Source: CAD feature listing. Evaluate the final solid. Frame: model axes, mm. A direction names the side the tool comes from. Coordinates: 2 decimals unless noted, no trailing zeros. Write each loop counter-clockwise with the first axis right and the second up, starting at its lowest first coordinate (ties: lowest second). Pieces come first, ordered by that corner, then holes. Notation, with made-up numbers: (40, 13) -> (57, 13) arc R22 cw to (57, 26) -> close; hole circle Ø10 at (69.5, 45.5). An arc over 180 degrees is marked (long way). Write item = value, one per line.
from build123d import *

# Parameters (mm, degrees)
BOSS_EXTRUDE1_DEPTH = 115.8875
CUT_EXTRUDE1_REACH  = 194.846
SKETCH3_W           = 213.51875
SKETCH3_H           = 129.38125
CUT_EXTRUDE3_DEPTH  = 4.7625
FILLET1_R           = 3.175
CUT_EXTRUDE4_START  = -4.7625
CUT_EXTRUDE4_DEPTH  = 4.7625


with BuildPart() as part:
    # Sketch1 → Boss-Extrude1 (new, symmetric)
    with BuildSketch(Plane.XY):
        Polygon((0, 0), (65.143179844, 139.7), (65.143179844, 124.674619947), (7.006449785, 0), align=None)
    extrude(amount=BOSS_EXTRUDE1_DEPTH, both=True)

    # Sketch2 → Cut-Extrude1 (cut, up to next)
    with BuildSketch(Plane(origin=(0, 0, 0), x_dir=(0, 0, 1), z_dir=(-0.906307787036651, 0.42261826174069705, 0)), mode=Mode.PRIVATE) as cut_extrude1_sk1:
        with BuildLine():
            Line((-98.679, 15.944158686), (-98.679, 128.720158686))
            ThreePointArc((-98.679, 128.720158686), (-98.38142049, 129.438579176), (-97.663, 129.736158686))
            Line((-97.663, 129.736158686), (97.663, 129.736158686))
            ThreePointArc((97.663, 129.736158686), (98.38142049, 129.438579176), (98.679, 128.720158686))
            Line((98.679, 128.720158686), (98.679, 15.944158686))
            ThreePointArc((98.679, 15.944158686), (98.38142049, 15.225738197), (97.663, 14.928158686))
            Line((97.663, 14.928158686), (-97.663, 14.928158686))
            ThreePointArc((-97.663, 14.928158686), (-98.38142049, 15.225738197), (-98.679, 15.944158686))
        make_face()
    cut_extrude1_tool1 = extrude(cut_extrude1_sk1.sketch, amount=-CUT_EXTRUDE1_REACH, mode=Mode.PRIVATE) & part.part
    add(cut_extrude1_tool1.solids().sort_by_distance((30.568891, 65.555199, 0))[0], mode=Mode.SUBTRACT)

    # Sketch3 → Cut-Extrude3 (cut)
    with BuildSketch(Plane(origin=(5.755054448, -2.683625962, 0), x_dir=(0, 0, -1), z_dir=(0.906307787036651, -0.42261826174069717, 0))):
        with Locations((-0.396875, 73.519608686)):
            Rectangle(SKETCH3_W, SKETCH3_H)
    extrude(amount=-CUT_EXTRUDE3_DEPTH, mode=Mode.SUBTRACT)

    # Fillet1
    fillet1_edges = [part.edges().sort_by_distance(p)[0] for p in [
        (7.328198768, 6.32451044, 107.15625),
        (62.007077745, 123.583744812, 107.15625),
        (62.007077745, 123.583744812, -106.3625),
        (7.328198768, 6.32451044, -106.3625),
    ]]
    fillet(fillet1_edges, radius=FILLET1_R)

    # Sketch4 → Cut-Extrude4 (cut)
    with BuildSketch(Plane(origin=(5.755054448, -2.683625962, 0), x_dir=(0, 0, -1), z_dir=(0.906307787036651, -0.42261826174069717, 0)).offset(CUT_EXTRUDE4_START)):
        with BuildLine():
            Line((107.95, 12.003983686), (107.95, 135.035233686))
            ThreePointArc((107.95, 135.035233686), (106.555096045, 138.402829732), (103.1875, 139.797733686))
            Line((103.1875, 139.797733686), (-103.98125, 139.797733686))
            ThreePointArc((-103.98125, 139.797733686), (-107.348846045, 138.402829732), (-108.74375, 135.035233686))
            Line((-108.74375, 135.035233686), (-108.74375, 12.003983686))
            ThreePointArc((-108.74375, 12.003983686), (-107.348846045, 8.636387641), (-103.98125, 7.241483686))
            Line((-103.98125, 7.241483686), (103.1875, 7.241483686))
            ThreePointArc((103.1875, 7.241483686), (106.555096045, 8.636387641), (107.95, 12.003983686))
        make_face()
        with BuildLine():
            Line((-103.98125, 8.828983686), (103.1875, 8.828983686))
            ThreePointArc((103.1875, 8.828983686), (105.43256403, 9.758919656), (106.3625, 12.003983686))
            Line((106.3625, 12.003983686), (106.3625, 135.035233686))
            ThreePointArc((106.3625, 135.035233686), (105.43256403, 137.280297717), (103.1875, 138.210233686))
            Line((103.1875, 138.210233686), (-103.98125, 138.210233686))
            ThreePointArc((-103.98125, 138.210233686), (-106.22631403, 137.280297717), (-107.15625, 135.035233686))
            Line((-107.15625, 135.035233686), (-107.15625, 12.003983686))
            ThreePointArc((-107.15625, 12.003983686), (-106.22631403, 9.758919656), (-103.98125, 8.828983686))
        make_face(mode=Mode.SUBTRACT)
    extrude(amount=CUT_EXTRUDE4_DEPTH, mode=Mode.SUBTRACT)


solid = part.part
1) Reachability of faces 4 (the flat face through (8.22, 2.6, 0.54)), 5 (the cylindrical face through (7.232, 6.198, 107.386)), 6 (the flat face through (5.67, 8.4, 0.9)), 7 (the cylindrical face through (62.04, 123.74, -106.59)) from +Z, -Z, +X, -X, +Y, -Y: full face, straight path, thin tool, end or side. Return the list, or none.
Answer block:
face_4 = +Z, -Z, +X, -Y
face_5 = +X
face_6 = none
face_7 = -Y
2) First-contact query: pin 1 Ø2 at (x, z) = (8, 21) entering from +Y. Flat tip, straight axial feed; report the tip coordinate or a pass-through.
Answer block:
pin_1 = 13.21
3) Cut plane C-C, the plane y = 129. Output: boundary loops of the cut face in (x, z).
Answer block:
outline = (60.15, -115.89) -> (65.14, -115.89) -> (65.14, 115.89) -> (60.15, 115.89) -> close
4) Material intervals for probe 1 along Z at (x, y) = (31.5, 57.5); probe 2 along Y at (x, z) = (7.5, 91); probe 3 along X at (y, z) = (127, 86), sorted ascending. Write a range as [from, to].
Answer block:
probe_1 = [-115.89, -107.95], [108.74, 115.89]
probe_2 = [1.06, 4.49], [12.33, 12.97]
probe_3 = [59.22, 65.14]
5) Pull-direction query (X, two-part tool) for faces 1 (the flat face through (61.068, 130.961, 1.622)), 2 (the flat face through (35, 65, 115.888)), 3 (the flat face through (62.648, 125.037, -1.053)); classes: +X half, -X half, draft (parallel to the pull), parting line (faces both ways), or undercut.
Answer block:
face_1 = -X half
face_2 = draft
face_3 = undercut
6) Cut plane A-A, the plane z = -83. Output: boundary loops of the cut face in (x, y).
Answer block:
outline = (0, 0) -> (7.01, 0) -> (8.82, 3.88) -> (4.5, 5.89) -> (7.75, 12.86) -> (6.31, 13.53) -> close; (54.83, 117.58) -> (56.27, 116.91) -> (60.52, 126.03) -> (64.84, 124.02) -> (65.14, 124.67) -> (65.14, 139.7) -> close
7) Cut plane B-B, the plane x = 17. Output: boundary loops of the cut face in (y, z).
Answer block:
outline = (21.43, -115.89) -> (36.46, -115.89) -> (36.46, -98.68) -> (32.7, -98.68) -> (32.7, -107.95) -> (21.43, -107.95) -> close; (21.43, 108.74) -> (32.7, 108.74) -> (32.7, 98.68) -> (36.46, 98.68) -> (36.46, 115.89) -> (21.43, 115.89) -> close
